from build123d import *

# Parameters (mm, degrees)
F3_START = 5.05
F3_DEPTH = 1.2


with BuildPart() as f1:
    # F0 (on Front) → F1 (revolve)
    with BuildSketch(Plane.XZ):
        Polygon((0, 11.15), (0, 4), (17, 4), (17, 11.15), (16, 11.15), (16, 4.75), (1, 4.75), (1, 11.15), align=None)
    revolve(axis=Axis((9.8618045449, 0, 0), (-1, 0, 0)))

    # F2 (on Front) → F3 (join)
    with BuildSketch(Plane.XZ.offset(F3_START)):
        with BuildLine():
            Line((17, 5.75), (17, -5.75))
            ThreePointArc((17, -5.75), (18, 0), (17, 5.75))
        make_face()
    extrude(amount=F3_DEPTH)


solid = f1.part
Check sheet for the modelled part. Datum: model origin and axes. Units: mm. A direction names the side the tool comes from. Round coordinates to 2 decimals unless told otherwise and drop trailing zeros. Order: outer loops, then holes, each group sorted by start corner. A loop starts at its lowest first (then second) coordinate and runs counter-clockwise, first axis right, second up. Notation, with made-up numbers: M -16.5,-4 L -4.5,-4 A13 ccw -4.5,10 Z; hole C -14.75,-32.75 d7. An arc over 180 degrees is marked long. One line per item, written item: value. Start each with the question number.
1. Section check B-B on z = 0. Enter the section's corners in (x, y).
2. Section check D-D on x = 16.5. Enter the section's corners in (y, z).
3. Access from +Z, -Z, +X, -X, +Y, -Y to the whole of each face (thin tool, end or side, straight path). Record for faces 4 (the flat face through (17.4, -6.25, 0.1)), 5 (the flat face through (17.4, -5.05, 0.1)), 6 (the flat face through (16, -5, 0)).
4. Section check C-C on y = -7. Enter the section's corners in (x, z).
5. Release check for a two-part mould opening along Z. For faces 1 (the cylindrical face through (16.493, 3.349, 10.635)), 2 (the flat face through (17, -4.8, 0.2)), 3 (the cylindrical face through (8.619, -3.905, -0.867)) record: released by +Z, released by -Z, zero draft, split by the parting line, or undercut.
6. Section check A-A on y = 6. Enter the section's corners in (x, z), and give its area (3 significant figures).
7. Scan lines: line 1 along X through (y, z) = (-7.5, -2.75); line 2 along Y through (x, z) = (9.5, 0); line 3 along Y through (x, z) = (15.5, 0.75). Record each from-to range of solid material in increasing order.
8. Gauge pin test, flat ends, axial feed: P1, Ø6, axis at x = 12.5, z = 1, coming from the -Y side; P2, Ø12, axis at y = 3, z = -5, coming from the +X side; P3, Ø4, axis at x = 9, z = 3, coming from the +Y side; P4, Ø6.5, axis at y = 0, z = 0, coming from the +X side. Record the tip position at first contact, or that the pin passes through.
Results found:
1. outline: M 0,-11.15 L 1,-11.15 L 1,-4.75 L 16,-4.75 L 16,-11.15 L 17,-11.15 L 17,-6.25 L 18,-6.25 L 18,-5.05 L 17,-5.05 L 17,-4 L 0,-4 Z; M 0,4 L 17,4 L 17,11.15 L 16,11.15 L 16,4.75 L 1,4.75 L 1,11.15 L 0,11.15 Z
2. outline: C 0,0 d22.3; hole C 0,0 d8
3. face 4: +Z, -Z, +X, -Y
3. face 5: +Z, -Z, +X, +Y
3. face 6: none
4. outline: M 0,-8.68 L 1,-8.68 L 1,8.68 L 0,8.68 Z; M 16,-8.68 L 17,-8.68 L 17,8.68 L 16,8.68 Z
5. face 1: split by the parting line
5. face 2: zero draft
5. face 3: undercut
6. outline: M 0,-9.4 L 1,-9.4 L 1,9.4 L 0,9.4 Z; M 16,-9.4 L 17,-9.4 L 17,9.4 L 16,9.4 Z
6. area: 37.6 mm^2
7. line 1: 0 to 1, 16 to 17
7. line 2: -4.75 to -4, 4 to 4.75
7. line 3: -4.69 to -3.93, 3.93 to 4.69
8. P1: y = -4.75
8. P2: x = 17
8. P3: y = 4.64
8. P4: through
